Check sheet for the modelled part. Datum: model origin and axes. Units: mm. Face numbers are marked on the shaded views. A direction names the side the tool comes from. Coordinates: 2 decimals unless noted, no trailing zeros. Write each loop counter-clockwise with the first axis right and the second up, starting at its lowest first coordinate (ties: lowest second). Pieces come first, ordered by that corner, then holes. Notation, with made-up numbers: (-4, 23) -> (8, 23) arc R14 ccw to (8, 29) -> close; hole circle Ø1 at (-36, 55.25). An arc over 180 degrees is marked (long way). One line per item, written item: value. Start each with the question number.
1) Draft check along Z on the marked faces 4 and 5. Enter one of: +Z half, -Z half, draft (parallel to the pull), parting line (faces both ways), or undercut.
2) Sectioned sample at D-D on z = -149. Enter the section's corners in (x, y).
3) Gauge pin test, flat ends, axial feed: P1, Ø6.5, axis at x = -11, z = -73, coming from the +Y side; P2, Ø3, axis at x = -12.5, z = -138.5, coming from the -Y side; P3, Ø6, axis at x = -8, z = -84, coming from the -Y side; P4, Ø10, axis at y = 18.5, z = -124.5, coming from the -X side. Record the tip position at first contact, or that the pin passes through.
4) Sectioned sample at A-A on y = 13.5. Enter the section's corners in (x, z).
5) Set-up check for the marked faces 1, 2 and 3: record each of +Z, -Z, +X, -X, +Y, -Y from which the full face is reachable in a straight line by a thin tool's end or side.
6) Sectioned sample at C-C on x = -5.75. Enter the section's corners in (y, z) (3 decimals).
7) Sectioned sample at B-B on y = 0. Enter the section's corners in (x, z), plus the area to 3 significant figures.
8) Scan lines: line 1 along X through (y, z) = (-9, -136); line 2 along Y through (x, z) = (-13, -46); line 3 along Z through (x, y) = (-8.75, -14). Record each from-to range of solid material in increasing order. Write a range as [from, to].
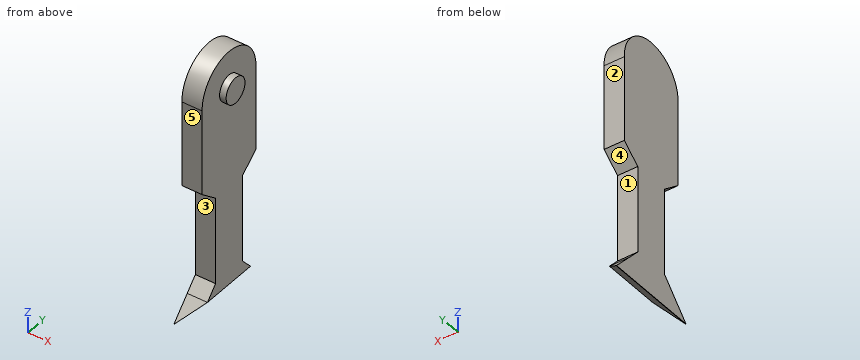
```python
from build123d import *

# Parameters (mm, degrees)
F0_R     = 8.255
F1_DEPTH = 4.189812
F3_DEPTH = 12.934547
F4_SIZE  = 12.7


with BuildPart() as f1:
    # F0 (on Right) → F1 (new body)
    with BuildSketch(Plane.YZ):
        with Locations((0, -36.195)):
            Circle(F0_R)
    extrude(amount=-F1_DEPTH)

    # F2 (on face) → F3 (join)
    with BuildSketch(Plane(origin=(-4.189812, 0, 0), x_dir=(0, -1, 0), z_dir=(-1, 0, 0))):
        with BuildLine():
            ThreePointArc((23.570169, -36.736008), (0, -12.618623), (-23.570169, -36.736008))
            Line((-23.570169, -36.736008), (-23.570169, -91.458903))
            Line((-23.570169, -91.458903), (-11.775727, -101.195575))
            Line((-11.775727, -101.195575), (-11.775727, -157.075575))
            Line((-11.775727, -157.075575), (-18.880744, -164.907241))
            Line((-18.880744, -164.907241), (-30.402395, -177.607241))
            Line((-30.402395, -177.607241), (30.402395, -177.607241))
            Line((30.402395, -177.607241), (18.880744, -164.907241))
            Line((18.880744, -164.907241), (11.775727, -157.075575))
            Line((11.775727, -157.075575), (11.775727, -101.195575))
            Line((11.775727, -101.195575), (23.570169, -91.458903))
            Line((23.570169, -91.458903), (23.570169, -36.736008))
        make_face()
    extrude(amount=F3_DEPTH)

    # F4
    f4_edges = [f1.edges().sort_by_distance(p)[0] for p in [
        (-4.189812, 0, -177.607241),
    ]]
    chamfer(f4_edges, length=F4_SIZE)


solid = f1.part
```
Answers:
1. face 4: undercut
1. face 5: draft
2. outline: (-17.12, -11.78) -> (-4.19, -11.78) -> (-4.19, 11.78) -> (-17.12, 11.78) -> close
3. P1: stops at y = 23.57
3. P2: stops at y = -11.78
3. P3: stops at y = -23.57
3. P4: passes through
4. outline: (-17.12, -177.61) -> (-16.89, -177.61) -> (-4.19, -164.91) -> (-4.19, -158.98) -> (-17.12, -158.98) -> close; (-17.12, -99.77) -> (-4.19, -99.77) -> (-4.19, -16.87) -> (-17.12, -16.87) -> close
5. face 1: +X, -X, +Y
5. face 2: +Z, +X, -X, +Y
5. face 3: +X, -X, -Y
6. outline: (-23.57, -91.459) -> (-11.776, -101.196) -> (-11.776, -157.076) -> (-20.296, -166.467) -> (20.296, -166.467) -> (11.776, -157.076) -> (11.776, -101.196) -> (23.57, -91.459) -> (23.57, -36.736) arc R23.576 ccw (long way) to (-23.57, -36.736) -> close
7. outline: (-17.12, -177.61) -> (-16.89, -177.61) -> (-4.19, -164.91) -> (-4.19, -44.45) -> (0, -44.45) -> (0, -27.94) -> (-4.19, -27.94) -> (-4.19, -12.62) -> (-17.12, -12.62) -> close
7. area: 2,120 mm2
8. line 1: x = [-17.12, -4.19]
8. line 2: y = [-23.57, 23.57]
8. line 3: z = [-169.47, -159.53], [-99.36, -17.23]
